The drawing under review shows one solid part. Ordinate dimensions are in mm from its lowest x, y, z. A direction names the side the tool comes from. Give positions to 0.01 mm unless a question says otherwise; leave off trailing zeros. Write each loop counter-clockwise with the first axis right and the second up, starting at its lowest first coordinate (ties: lowest second). Pieces come first, ordered by that corner, then holes. Notation, with made-up numbers: (64, 7.5) -> (102, 7.5) arc R25 ccw to (102, 33.5) -> close; hole circle Ø4 at (-17, -26.5). An arc over 180 degrees is marked (long way). Write item = value, one per line.
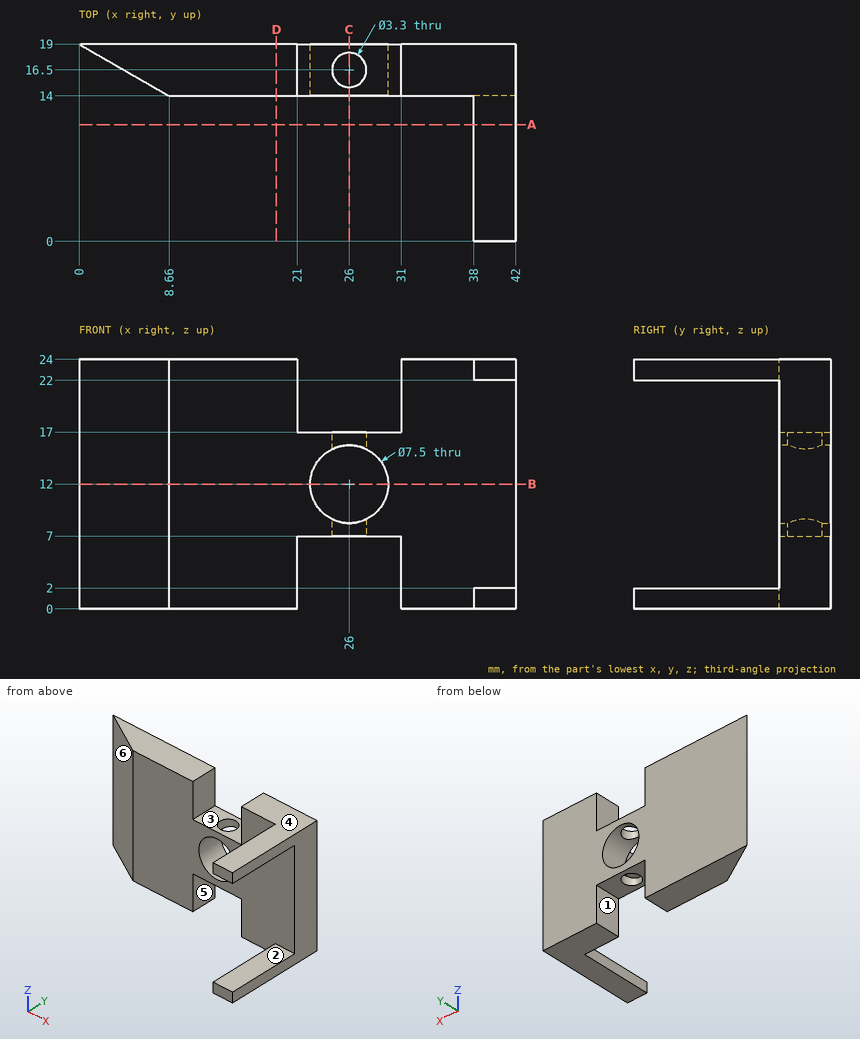
(1) Take a section at A-A (y = 11.25). Write out the cut boundary in (x, z).
Answers below:
outline = (38, 0) -> (42, 0) -> (42, 2) -> (38, 2) -> close; (38, 22) -> (42, 22) -> (42, 24) -> (38, 24) -> close
(2) Take a section at B-B (z = 12). Write out the cut boundary in (x, y), plus the area to 3 significant figures.
Answers below:
outline = (0, 19) -> (8.66, 14) -> (22.25, 14) -> (22.25, 19) -> close; (29.75, 14) -> (42, 14) -> (42, 19) -> (29.75, 19) -> close
area = 151 mm^2
(3) To check wall thickness, follow probe 1 along Y at (x, z) = (26, 7.9); probe 2 along Y at (x, z) = (38, 5.5); probe 3 along X at (y, z) = (16.5, 15.85). State the ranges of each line that lie inside material, in increasing order.
Answers below:
probe_1 = 14 to 14.85, 18.15 to 19
probe_2 = 14 to 19
probe_3 = 4.33 to 24.35, 27.65 to 42
(4) Take a section at C-C (x = 26). Write out the cut boundary in (y, z).
Answers below:
outline = (14, 7) -> (14.85, 7) -> (14.85, 8.25) -> (14, 8.25) -> close; (14, 15.75) -> (14.85, 15.75) -> (14.85, 17) -> (14, 17) -> close; (18.15, 7) -> (19, 7) -> (19, 8.25) -> (18.15, 8.25) -> close; (18.15, 15.75) -> (19, 15.75) -> (19, 17) -> (18.15, 17) -> close
(5) For pin 1 (4 mm diameter, centred on y = 13, z = 14, fed in from +X); pin 2 (5.5 mm diameter, centred on x = 26, y = 16.5, fed in from +Z); pin 3 (1.6 mm diameter, centred on y = 5.5, z = 1, fed in from -X); pin 4 (7 mm diameter, centred on x = 20, z = 16.5, fed in from -Y), all flat-tipped, find the tip position at first contact; note any pin that passes through.
Answers below:
pin_1 = 42
pin_2 = 17
pin_3 = 38
pin_4 = 14
(6) Tool access review of the marked faces 1, 2 and 3: name each direction out of +Z, -Z, +X, -X, +Y, -Y from which nothing blocks a thin tool from reaching the whole face with its end or side.
Answers below:
face_1 = -Z, +Y, -Y
face_2 = +X, -X, -Y
face_3 = +Z, +Y, -Y
(7) Take a section at D-D (x = 19). Write out the cut boundary in (y, z), plus the area to 3 significant figures.
Answers below:
outline = (14, 0) -> (19, 0) -> (19, 24) -> (14, 24) -> close
area = 120 mm^2
(8) The part is to be moulded in two halves that separate along X. For the marked faces 4, 5 and 6, say which applies: released by +X, released by -X, zero draft, split by the parting line, or undercut.
Answers below:
face_4 = zero draft
face_5 = undercut
face_6 = released by -X
